Can you work these out from the drawing? Everything is in mm from the part's minimum corner. Round coordinates to 2 decimals unless told otherwise and drop trailing zeros. Order: outer loops, then holes, each group sorted by start corner. A loop starts at its lowest first (then second) coordinate and runs counter-clockwise, first axis right, second up. Notation, with made-up numbers: (-27, -14.5) -> (13, -14.5) arc R20 cw to (13, 19.5) -> close; hole circle Ø8 at (49.5, 88). An arc over 180 degrees is marked (long way). One line per item, written item: value.
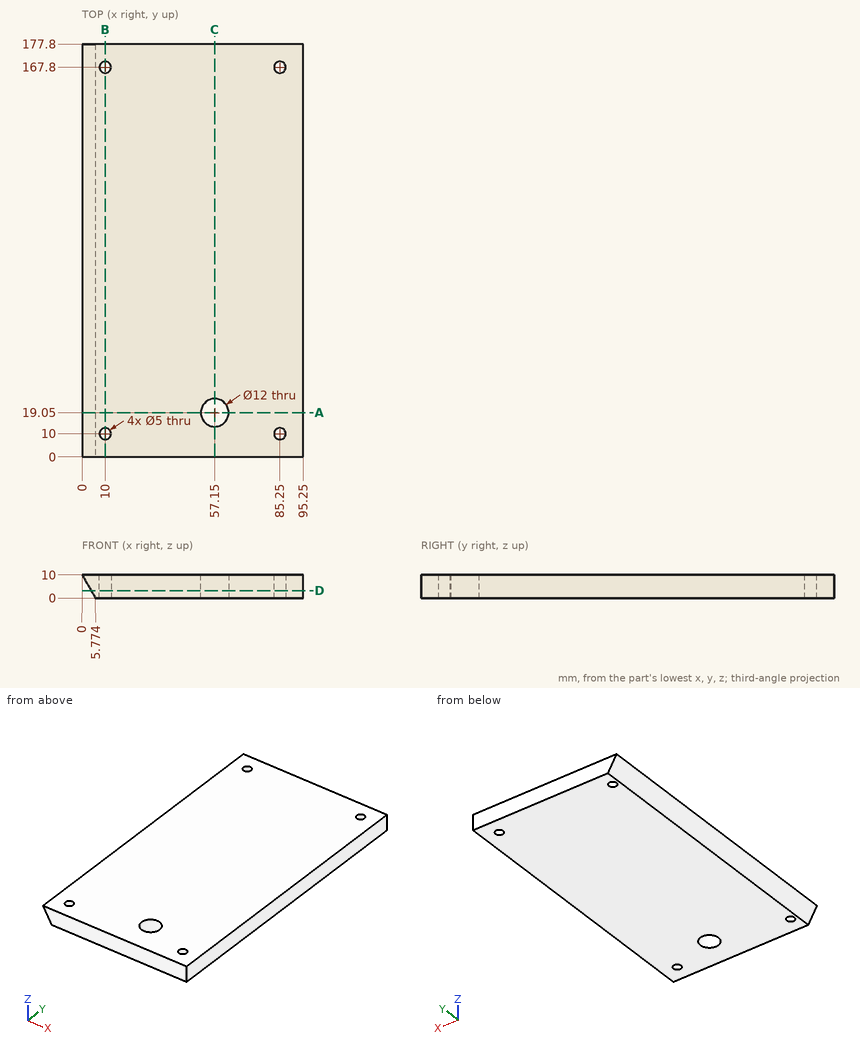
Q1. For P1, Ø1.5, axis at y = 79, z = 4, coming from the -X side; P2, Ø2, axis at y = 125, z = 5.5, coming from the -X side, each with a flat end and sliding along its axis, tell me the tip position at first contact or that it passes through.
Answers:
P1: x = 3.03
P2: x = 2.02
Q2. I need wall thicknesses on line 1 along Y through (x, z) = (10, 3.5); line 2 along Y through (x, z) = (56.5, 5.75) (1 decimal); line 3 along Y through (x, z) = (56, 6.25). Which ranges of each line are inside material? Lowest first, please.
Answers:
line 1: 0 to 7.5, 12.5 to 165.3, 170.3 to 177.8
line 2: 0 to 13.1, 25 to 177.8
line 3: 0 to 13.16, 24.94 to 177.8
Q3. I want a section at B-B on x = 10. Write out the boundary of the cut face in (y, z), then the cut area to 3 significant figures.
Answers:
outline: (0, 0) -> (7.5, 0) -> (7.5, 10) -> (0, 10) -> close; (12.5, 0) -> (165.3, 0) -> (165.3, 10) -> (12.5, 10) -> close; (170.3, 0) -> (177.8, 0) -> (177.8, 10) -> (170.3, 10) -> close
area: 1,680 mm2
Q4. I want a section at C-C on x = 57.15. Write out the boundary of the cut face in (y, z), then the cut area to 3 significant figures.
Answers:
outline: (0, 0) -> (13.05, 0) -> (13.05, 10) -> (0, 10) -> close; (25.05, 0) -> (177.8, 0) -> (177.8, 10) -> (25.05, 10) -> close
area: 1,660 mm2
Q5. I want a section at D-D on z = 3.25. Write out the boundary of the cut face in (x, y), then the cut area to 3 significant figures.
Answers:
outline: (3.9, 0) -> (95.25, 0) -> (95.25, 177.8) -> (3.9, 177.8) -> close; hole circle Ø5 at (10, 10); hole circle Ø5 at (10, 167.8); hole circle Ø12 at (57.15, 19.05); hole circle Ø5 at (85.25, 10); hole circle Ø5 at (85.25, 167.8)
area: 16,100 mm2
Q6. I want a section at A-A on y = 19.05. Write out the boundary of the cut face in (x, z).
Answers:
outline: (0, 10) -> (5.77, 0) -> (51.15, 0) -> (51.15, 10) -> close; (63.15, 0) -> (95.25, 0) -> (95.25, 10) -> (63.15, 10) -> close
